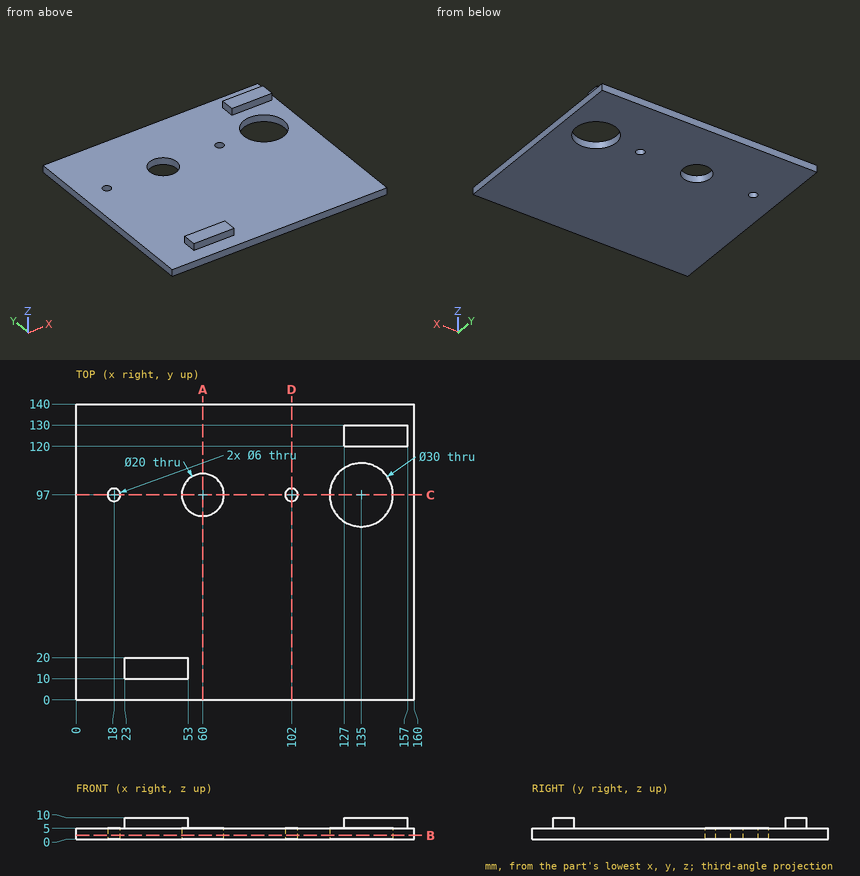
Geometry check sheet. Reference: drawing and pictorial views, mm from the part's lowest x, y, z. Coordinates: 2 decimals unless noted, no trailing zeros. Order: outer loops, then holes, each group sorted by start corner. A loop starts at its lowest first (then second) coordinate and runs counter-clockwise, first axis right, second up. Notation, with made-up numbers: M 46.5,-32 L 71.5,-32 A21 ccw 71.5,-23 Z; hole C 86,88.5 d7. An arc over 180 degrees is marked long. Return JSON: item names as keys, results as strings.
1) Cross-section at A-A, the plane x = 60. Record the boundary of the cut face in (y, z).
Answer list:
{"outline": "M 0,0 L 87,0 L 87,5 L 0,5 Z; M 107,0 L 140,0 L 140,5 L 107,5 Z"}
2) Thickness scan on L1, parallel to X at y = 97, z = 1.45; L2, parallel to Y at x = 135, z = 3.7; L3, parallel to Y at x = 60, z = 2.6. Record the ranges inside material, lowest first. Write a range as [from, to].
Answer list:
{"L1": "[0, 15], [21, 50], [70, 99], [105, 120], [150, 160]", "L2": "[0, 82], [112, 140]", "L3": "[0, 87], [107, 140]"}
3) Gauge pin test, flat ends, axial feed: pin 1 (4 mm diameter, centred on x = 136.5, z = 7.5, fed in from +Y); pin 2 (2.5 mm diameter, centred on x = 35.5, z = 8.5, fed in from -Y); pin 3 (1.5 mm diameter, centred on x = 135.5, z = 8, fed in from -Y). Record the tip position at first contact, or that the pin passes through.
Answer list:
{"pin 1": "y = 130", "pin 2": "y = 10", "pin 3": "y = 120"}
4) Cross-section at C-C, the plane y = 97. Record the boundary of the cut face in (x, z), and give its area (3 significant figures).
Answer list:
{"outline": "M 0,0 L 15,0 L 15,5 L 0,5 Z; M 21,0 L 50,0 L 50,5 L 21,5 Z; M 70,0 L 99,0 L 99,5 L 70,5 Z; M 105,0 L 120,0 L 120,5 L 105,5 Z; M 150,0 L 160,0 L 160,5 L 150,5 Z", "area": "490 mm2"}
5) Cross-section at D-D, the plane x = 102. Record the boundary of the cut face in (y, z), and give its area (3 significant figures).
Answer list:
{"outline": "M 0,0 L 94,0 L 94,5 L 0,5 Z; M 100,0 L 140,0 L 140,5 L 100,5 Z", "area": "670 mm2"}
6) Cross-section at B-B, the plane z = 1.75. Record the boundary of the cut face in (x, y).
Answer list:
{"outline": "M 0,0 L 160,0 L 160,140 L 0,140 Z; hole C 18,97 d6; hole C 60,97 d20; hole C 102,97 d6; hole C 135,97 d30"}
